The listing builds one solid part. Answer for the finished solid, in the listing's coordinates (mm). Face numbers are marked on the shaded views. A direction names the side the tool comes from. Give positions to 0.01 mm unless a question says otherwise; leave off trailing zeros. Order: outer loops, then holes, each group sorted by start corner. A loop starts at its lowest first (then second) coordinate and runs counter-clockwise, first axis right, second up. Notation, with made-up numbers: (11, -26.5) -> (69, -26.5) arc R16 cw to (69, -4.5) -> close; hole circle Ø6 at (85, 72). An arc over 180 degrees is marked (long way). Write item = value, one per line. Start each with the question number.
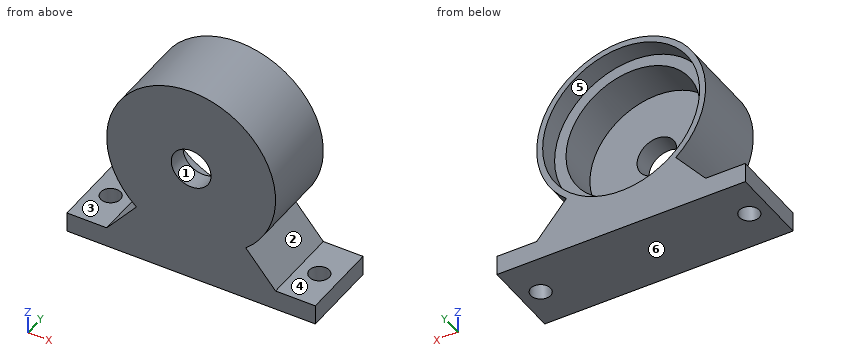
```python
from build123d import *

# Parameters (mm, degrees)
SKETCH_1_R          = 8
SKETCH_1_R_2        = 6.75
EXTRUDE_2_DEPTH     = 6
SKETCH_2_R          = 6.75
SKETCH_2_R_2        = 2
EXTRUDE_3_DEPTH     = 2
SKETCH_3_R          = 8.5
SKETCH_3_R_2        = 7.9
EXTRUDE_4_DEPTH     = 2
SKETCH_4_R          = 8.5
SKETCH_4_R_2        = 8
EXTRUDE_6_DEPTH     = 6
EXTRUDE_8_DEPTH     = 8
SKETCH_7_R          = 1
CUT_EXTRUDE_1_DEPTH = 8


with BuildPart() as part:
    # 草图1 → 凸台-拉伸2 (new body)
    with BuildSketch(Plane(origin=(0, 0, 0), x_dir=(1, 0, 0), z_dir=(0, 1, 0))):
        Circle(SKETCH_1_R)
        Circle(SKETCH_1_R_2, mode=Mode.SUBTRACT)
    extrude(amount=EXTRUDE_2_DEPTH)

    # 草图2 → 凸台-拉伸3 (add)
    with BuildSketch(Plane(origin=(0, 0, 0), x_dir=(1, 0, 0), z_dir=(0, 1, 0))):
        Circle(SKETCH_2_R)
        Circle(SKETCH_2_R_2, mode=Mode.SUBTRACT)
    extrude(amount=EXTRUDE_3_DEPTH)

    # 草图3 → 凸台-拉伸4 (add)
    with BuildSketch(Plane(origin=(0, 6, 0), x_dir=(1, 0, 0), z_dir=(0, 1, 0))):
        Circle(SKETCH_3_R)
        Circle(SKETCH_3_R_2, mode=Mode.SUBTRACT)
    extrude(amount=EXTRUDE_4_DEPTH)

    # 草图4 → 凸台-拉伸6 (add)
    with BuildSketch(Plane.XZ.offset(-6)):
        Circle(SKETCH_4_R)
        Circle(SKETCH_4_R_2, mode=Mode.SUBTRACT)
    extrude(amount=EXTRUDE_6_DEPTH)

    # 草图6 → 凸台-拉伸8 (add)
    with BuildSketch(Plane.XZ):
        with BuildLine():
            Line((-8.5, -10), (-5.505011571, -6.476484201))
            ThreePointArc((-5.505011571, -6.476484201), (0, -8.5), (5.505011571, -6.476484201))
            Line((5.505011571, -6.476484201), (8.5, -10))
            Line((8.5, -10), (12.5, -10))
            Line((12.5, -10), (12.5, -12))
            Line((12.5, -12), (0, -12))
            Line((0, -12), (-12.5, -12))
            Line((-12.5, -12), (-12.5, -10))
            Line((-12.5, -10), (-8.5, -10))
        make_face()
    extrude(amount=-EXTRUDE_8_DEPTH)

    # 草图7 → 切除-拉伸1 (cut)
    with BuildSketch(Plane(origin=(0, 0, -12), x_dir=(-1, 0, 0), z_dir=(0, 0, -1))):
        with Locations((10.5, 4)):
            Circle(SKETCH_7_R)
        with Locations((-10.5, 4)):
            Circle(SKETCH_7_R)
    extrude(amount=-CUT_EXTRUDE_1_DEPTH, mode=Mode.SUBTRACT)


solid = part.part
```
Item 1: A cutting plane is placed at A-A, the plane x = 0. Write down the section's boundary in (y, z).
Item 2: The mould has two halves that part along X. Classify the marked faces 1, 2 and 3: +X half, -X half, draft (parallel to the pull), parting line (faces both ways), or undercut.
Item 3: A cutting plane is placed at C-C, the plane z = 0. Write down the section's boundary in (x, y).
Item 4: A cutting plane is placed at D-D, the plane y = 1. Write down the section's boundary in (x, z), plus the area to 3 significant figures.
Item 5: Which of the six approach directions +Z, -Z, +X, -X, +Y, -Y give full straight-line access (tool end or side, diameter ignored) to the marked faces 4, 5 and 6?
Item 6: A cutting plane is placed at B-B, the plane y = 4. Write down the section's boundary in (x, z), plus the area to 3 significant figures.
Item 7: Consider L1, parallel to X at y = 7.35, z = 0; L2, parallel to Y at x = -10.5, z = -10.7; L3, parallel to Z at x = -5.75, y = 4.75. Determine where each line is inside the solid, lowest interval first. Write a range as from..to.
Item 8: Flat-ended cylindrical pins translate along their axes: pin 1 (12 mm diameter, centred on x = 0, z = 0, fed in from +Y); pin 2 (1.5 mm diameter, centred on y = 3, z = -4, fed in from -X); pin 3 (2.5 mm diameter, centred on x = 0, z = 0, fed in from -Y); pin 4 (1.5 mm diameter, centred on y = 5.5, z = -7, fed in from +X). Find the tip coordinate at first contact, or state that the pin passes through.
Check values:
q1.outline = (0, -12) -> (8, -12) -> (8, -7.9) -> (6, -7.9) -> (6, -6.75) -> (2, -6.75) -> (2, -2) -> (0, -2) -> close; (0, 2) -> (2, 2) -> (2, 6.75) -> (6, 6.75) -> (6, 7.9) -> (8, 7.9) -> (8, 8.5) -> (0, 8.5) -> close
q2.face_1 = undercut
q2.face_2 = +X half
q2.face_3 = draft
q3.outline = (-8.5, 0) -> (-2, 0) -> (-2, 2) -> (-6.75, 2) -> (-6.75, 6) -> (-7.9, 6) -> (-7.9, 8) -> (-8.5, 8) -> close; (2, 0) -> (8.5, 0) -> (8.5, 8) -> (7.9, 8) -> (7.9, 6) -> (6.75, 6) -> (6.75, 2) -> (2, 2) -> close
q4.outline = (-12.5, -12) -> (12.5, -12) -> (12.5, -10) -> (8.5, -10) -> (5.51, -6.48) arc R8.5 ccw (long way) to (-5.51, -6.48) -> (-8.5, -10) -> (-12.5, -10) -> close; hole circle Ø4 at (0, 0)
q4.area = 299 mm^2
q5.face_4 = +Z, +X, +Y, -Y
q5.face_5 = +Y
q5.face_6 = -Z, +X, -X, +Y, -Y
q6.outline = (-12.5, -12) -> (-11.5, -12) -> (-11.5, -10) -> (-12.5, -10) -> close; (-9.5, -12) -> (9.5, -12) -> (9.5, -10) -> (8.5, -10) -> (5.51, -6.48) arc R8.5 ccw (long way) to (-5.51, -6.48) -> (-8.5, -10) -> (-9.5, -10) -> close; (11.5, -12) -> (12.5, -12) -> (12.5, -10) -> (11.5, -10) -> close; hole circle Ø13.5 at (0, 0)
q6.area = 160 mm^2
q7.L1 = -8.5..-7.9, 7.9..8.5
q7.L2 = 0..3, 5..8
q7.L3 = -12..-6.76, -6.26..-3.54, 3.54..6.26
q8.pin_1 = 2
q8.pin_2 = -7.85
q8.pin_3 = through
q8.pin_4 = 6.59
